The drawing under review shows one solid part. Ordinate dimensions are in mm from its lowest x, y, z. Coordinates: 2 decimals unless noted, no trailing zeros. Loops run counter-clockwise (first coordinate to the right, second up) from the corner with the lowest first, then second, coordinate; pieces in that order, holes last. Notation, with made-up numbers: (-39.75, -24) -> (-21.75, -24) arc R27 ccw to (-21.75, 6) -> close; hole circle Ø7 at (9, 88.25). An arc over 180 degrees is marked (long way). Use a Markdown table: item, result.
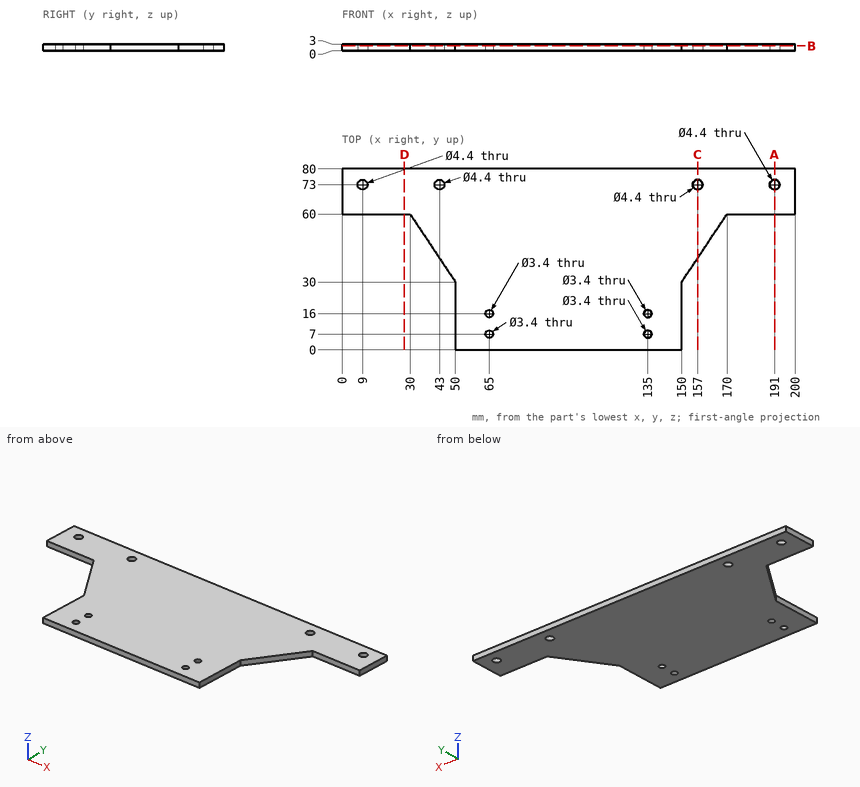
(1) Take a section at A-A on x = 191. Write out the cut boundary in (y, z).
Found:
| item | result |
|---|---|
| outline | (60, 0) -> (70.8, 0) -> (70.8, 3) -> (60, 3) -> close; (75.2, 0) -> (80, 0) -> (80, 3) -> (75.2, 3) -> close |
(2) For pin 1 Ø2 at (x, y) = (135, 7) entering from +Z; pin 2 Ø1.5 at (x, z) = (185.5, 2) entering from -Y; pin 3 Ø0.9 at (y, z) = (13, 1.5) entering from -X, all flat-tipped, find the tip position at first contact; note any pin that passes through.
Found:
| item | result |
|---|---|
| pin 1 | passes through |
| pin 2 | stops at y = 60 |
| pin 3 | stops at x = 50 |
(3) Take a section at C-C on x = 157. Write out the cut boundary in (y, z).
Found:
| item | result |
|---|---|
| outline | (40.5, 0) -> (70.8, 0) -> (70.8, 3) -> (40.5, 3) -> close; (75.2, 0) -> (80, 0) -> (80, 3) -> (75.2, 3) -> close |
(4) For line 1 along X through (y, z) = (7, 2.3); line 2 along Y through (x, z) = (65, 0.85); line 3 along X through (y, z) = (73, 2.2), list the stretches that pass through material, from the lowest coordinate up.
Found:
| item | result |
|---|---|
| line 1 | x = 50 to 63.3, 66.7 to 133.3, 136.7 to 150 |
| line 2 | y = 0 to 5.3, 8.7 to 14.3, 17.7 to 80 |
| line 3 | x = 0 to 6.8, 11.2 to 40.8, 45.2 to 154.8, 159.2 to 188.8, 193.2 to 200 |
(5) Take a section at B-B on z = 2.15. State how many separate pieces and enclosed holes the cut face has, plus the area to 3 significant figures.
Found:
| item | result |
|---|---|
| separate pieces | 1 |
| enclosed holes | 8 |
| area | 10,500 mm^2 |
(6) Take a section at D-D on x = 27.5. Write out the cut boundary in (y, z), plus the area to 3 significant figures.
Found:
| item | result |
|---|---|
| outline | (60, 0) -> (80, 0) -> (80, 3) -> (60, 3) -> close |
| area | 60.0 mm^2 |
